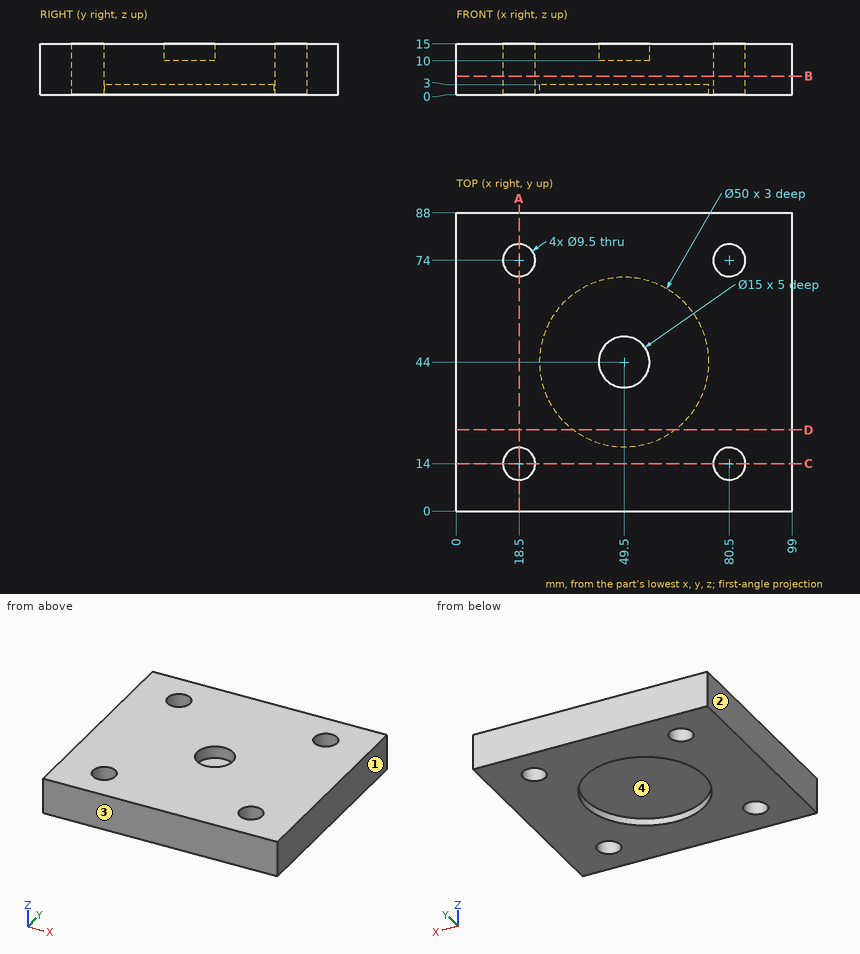
Study the drawing (mm; zero at the part's minimum x, y, z) and answer. Give positions to 0.01 mm unless a question says otherwise; leave off trailing zeros. Loops run counter-clockwise (first coordinate to the right, second up) from the corner with the lowest first, then second, coordinate; pieces in that order, holes last. Notation, with made-up numbers: (-5.5, 2) - (20.5, 2) arc R20 cw to (20.5, 32) - close; hole circle Ø11 at (89, 69). An arc over 180 degrees is marked (long way). Answer in a Markdown table with one row per item. Add a question column.
Q1. The part is cut by section C-C (y = 14). Determine the outline of the cut face in (x, z), and give its area (3 significant figures).
Q2. The part is cut by section D-D (y = 24). Determine the outline of the cut face in (x, z).
Q3. Consider line 1 along Y through (x, z) = (80.5, 10); line 2 along Y through (x, z) = (22.5, 0.75); line 3 along Y through (x, z) = (49.5, 2.2). Determine where each line is inside the solid, lowest interval first.
Q4. Determine the mould class of the marked faces 1, 2, 3 and 4 for opening direction X: released by +X, released by -X, zero draft, split by the parting line, or undercut.
Q5. The part is cut by section A-A (x = 18.5). Determine the outline of the cut face in (y, z).
Q6. Each of these flat-tipped pins is pushed along its axis until it touches: P1, Ø7.5, axis at x = 18.5, y = 14, coming from the -Z side; P2, Ø13.5, axis at x = 49.5, y = 44, coming from the -Z side. Where does it stop, or does it pass through?
Q7. The part is cut by section B-B (z = 5.5). Determine the outline of the cut face in (x, y).
Solution:
| question | item | result |
|---|---|---|
| 1 | outline | (0, 0) - (13.75, 0) - (13.75, 15) - (0, 15) - close; (23.25, 0) - (75.75, 0) - (75.75, 15) - (23.25, 15) - close; (85.25, 0) - (99, 0) - (99, 15) - (85.25, 15) - close |
| 1 | area | 1,200 mm² |
| 2 | outline | (0, 0) - (34.5, 0) - (34.5, 3) - (64.5, 3) - (64.5, 0) - (99, 0) - (99, 15) - (0, 15) - close |
| 3 | line 1 | y = 0 to 9.25, 18.75 to 69.25, 78.75 to 88 |
| 3 | line 2 | y = 0 to 11.44, 16.56 to 71.44, 76.56 to 88 |
| 3 | line 3 | y = 0 to 19, 69 to 88 |
| 4 | face 1 | released by +X |
| 4 | face 2 | released by -X |
| 4 | face 3 | zero draft |
| 4 | face 4 | undercut |
| 5 | outline | (0, 0) - (9.25, 0) - (9.25, 15) - (0, 15) - close; (18.75, 0) - (69.25, 0) - (69.25, 15) - (18.75, 15) - close; (78.75, 0) - (88, 0) - (88, 15) - (78.75, 15) - close |
| 6 | P1 | passes through |
| 6 | P2 | stops at z = 3 |
| 7 | outline | (0, 0) - (99, 0) - (99, 88) - (0, 88) - close; hole circle Ø9.5 at (18.5, 14); hole circle Ø9.5 at (18.5, 74); hole circle Ø9.5 at (80.5, 14); hole circle Ø9.5 at (80.5, 74) |
